```python
from build123d import *

# Parameters (mm, degrees)
SKETCH_R     = 1.2
PAD_DEPTH    = 3
PAD001_DEPTH = 10
FILLET_R     = 3
SKETCH002_R  = 2.5
POCKET_DEPTH = 6


with BuildPart() as part:
    # Sketch → Pad (new body)
    with BuildSketch(Plane.XY):
        Polygon((0, 12), (0, 0), (-20, 0), (-20, 12), (-15, 19.412805), (-5, 19.412805), align=None)
        with Locations((-13, 4)):
            Circle(SKETCH_R, mode=Mode.SUBTRACT)
        with Locations((-7, 4)):
            Circle(SKETCH_R, mode=Mode.SUBTRACT)
    extrude(amount=PAD_DEPTH)

    # Sketch001 (on Face10 of Pad) → Pad001 (join)
    with BuildSketch(Plane.XY.offset(3)):
        Polygon((-14.90374, 19.331674), (-5.09626, 19.331674), (-1.5, 14), (-18.5, 14), align=None)
    extrude(amount=PAD001_DEPTH)

    # Fillet
    fillet_edges = [part.edges().sort_by_distance(p)[0] for p in [
        (-3.29813, 16.665837, 13),
        (-10, 19.331674, 13),
        (-16.70187, 16.665837, 13),
    ]]
    fillet(fillet_edges, radius=FILLET_R)

    # Sketch002 (on Face12 of Pad001) → Pocket (cut)
    with BuildSketch(Plane.XZ.offset(-14)):
        with Locations((-10, 8)):
            Circle(SKETCH002_R)
    extrude(amount=-POCKET_DEPTH, mode=Mode.SUBTRACT)


solid = part.part
```
Check sheet for the modelled part. Datum: model origin and axes. Units: mm. A direction names the side the tool comes from. Round coordinates to 2 decimals unless told otherwise and drop trailing zeros. Order: outer loops, then holes, each group sorted by start corner. A loop starts at its lowest first (then second) coordinate and runs counter-clockwise, first axis right, second up.
1) Section check A-A (z = 8). Record the boundary of the cut face in (x, y).
2) Section check B-B (y = 4). Record the boundary of the cut face in (x, z), and give its area (3 significant figures).
3) Tool access check on faces 1 (the flat face through (-16.727, 16.629, 6.451)), 2 (the flat face through (-10, 19.332, 5)), 3 (the flat face through (-3.32, 16.7, 6.45)), 4 (the flat face through (-8, 14, 6)), 5 (the flat face through (-20, 6, 1)). Record the directions out of +Z, -Z, +X, -X, +Y, -Y that give a thin tool (end or side, any length) a straight path to the whole face; none if there is none.
4) Mould release check, pull along X, two halves, no side actions. Record for faces 6 (the cylindrical face through (-16.242, 16.41, 11.694)), 7 (the cylindrical face through (-9.931, 18.476, 12.098)), 8 (the cylindrical face through (-11.855, 4.36, 1.479)): +X half, -X half, draft (parallel to the pull), parting line (faces both ways), or undercut.
5) Section check C-C (x = -13). Record the boundary of the cut face in (y, z).
6) Section check D-D (z = 1.5). Record the boundary of the cut face in (x, y), and give its area (3 significant figures).
7) Go/stop test with flat-tipped pins: pin 1 Ø10 at (x, y) = (-5, 4.5) entering from -Z; pin 2 Ø5 at (x, z) = (-4, 8) entering from +Y; pin 3 Ø2 at (x, y) = (-2.5, 16.5) entering from +Z; pin 4 Ø6 at (x, y) = (-14.5, 6.5) entering from +Z. Record where each tip stops, or that it passes through.
8) Scan lines: line 1 (Y direction, x = -7, z = 0.95); line 2 (Z direction, x = -14.75, y = 5.25); line 3 (Y direction, x = -7, z = 9.5). Record each from-to range of solid material in increasing order.
Result:
1. outline: (-18.5, 14) - (-12.5, 14) - (-12.5, 19.33) - (-14.9, 19.33) - close; (-7.5, 14) - (-1.5, 14) - (-5.1, 19.33) - (-7.5, 19.33) - close
2. outline: (-20, 0) - (-14.2, 0) - (-14.2, 3) - (-20, 3) - close; (-11.8, 0) - (-8.2, 0) - (-8.2, 3) - (-11.8, 3) - close; (-5.8, 0) - (0, 0) - (0, 3) - (-5.8, 3) - close
2. area: 45.6 mm2
3. face 1: +Z, -X, +Y
3. face 2: +Z, +X, -X, +Y
3. face 3: +Z, +X, +Y
3. face 4: +Z, +X, -X, -Y
3. face 5: +Z, -Z, -X, +Y, -Y
4. face 6: -X half
4. face 7: draft
4. face 8: undercut
5. outline: (0, 0) - (2.8, 0) - (2.8, 3) - (0, 3) - close; (5.2, 0) - (19.41, 0) - (19.41, 3) - (19.33, 3) - (19.33, 10) arc R3 ccw to (16.33, 13) - (14, 13) - (14, 3) - (5.2, 3) - close
6. outline: (-20, 0) - (0, 0) - (0, 12) - (-5, 19.41) - (-15, 19.41) - (-20, 12) - close; hole circle Ø2.4 at (-13, 4); hole circle Ø2.4 at (-7, 4)
6. area: 342 mm2
7. pin 1: stops at z = 0
7. pin 2: stops at y = 19.33
7. pin 3: stops at z = 11.55
7. pin 4: stops at z = 3
8. line 1: y = 0 to 2.8, 5.2 to 19.41
8. line 2: z = 0 to 3
8. line 3: y = 14 to 19.33
